Check sheet for the modelled part. Datum: model origin and axes. Units: mm. A direction names the side the tool comes from. Coordinates: 2 decimals unless noted, no trailing zeros. Write each loop counter-clockwise with the first axis right and the second up, starting at its lowest first coordinate (ties: lowest second). Pieces come first, ordered by that corner, then holes. Notation, with made-up numbers: (18, 65) - (34, 65) arc R22 cw to (34, 98) - close; hole circle Ø1 at (46, 31.5). An arc over 180 degrees is marked (long way). Use one line per item in the form item = value. Start each with the question number.
1. Tool access check on faces 1 (the face through (-26, -26, 25)), 2 (the face through (-38, 24.325, 30)), 3 (the face through (-17.54, 37, 30)), 4 (the face through (-26, -30.675, 12)). Record the directions out of +Z, -Z, +X, -X, +Y, -Y that give a thin tool (end or side, any length) a straight path to the whole face; none if there is none.
2. Cross-section at D-D on x = -19. Record the boundary of the cut face in (y, z), then the cut area to 3 significant figures.
3. Draft check along Z on faces 5 (the face through (-26, -26, 35)), 6 (the face through (-0.54, 9, 30)), 7 (the face through (-26, -8, 60)). Enter one of: +Z half, -Z half, draft (parallel to the pull), parting line (faces both ways), or undercut.
4. Go/stop test with a flat-tipped pin: pin 1 Ø11 at (x, z) = (-29, 31.5) entering from -Y. Record where the tip stops, or that it passes through.
5. Cross-section at B-B on x = -35. Record the boundary of the cut face in (y, z).
6. Cross-section at C-C on z = 51.5. Record the boundary of the cut face in (x, y).
7. Cross-section at A-A on y = 27.5. Record the boundary of the cut face in (x, z).
8. Scan lines: line 1 along Y through (x, z) = (-16, 15); line 2 along X through (y, z) = (21.5, 43.5); line 3 along Z through (x, y) = (-14.5, -22.5). Record each from-to range of solid material in increasing order.
```python
from build123d import *

# Parameters (mm, degrees)
BOSS_EXTRUDE2_DEPTH = 60
SKETCH2_W           = 10
SKETCH2_H           = 10
CUT_EXTRUDE1_DEPTH  = 60


with BuildPart() as part:
    # Sketch1 → Boss-Extrude2 (new body)
    with BuildSketch(Plane.XY):
        Polygon((-50.540381022, -30.675149326), (-0.540381022, -30.675149326), (-0.540381022, 49.324850674), (-17.540381022, 49.324850674), (-17.540381022, 24.324850674), (-8.540381022, 24.324850674), (-8.540381022, -5.675149326), (-42.540381022, -5.675149326), (-42.540381022, 24.324850674), (-33.540381022, 24.324850674), (-33.540381022, 49.324850674), (-50.540381022, 49.324850674), align=None)
    extrude(amount=BOSS_EXTRUDE2_DEPTH)

    # Sketch2 → Cut-Extrude1 (cut)
    with BuildSketch(Plane.ZY.offset(50.540381022)):
        with Locations((30, -25.675149326)):
            Rectangle(SKETCH2_W, SKETCH2_H)
    extrude(amount=-CUT_EXTRUDE1_DEPTH, mode=Mode.SUBTRACT)


solid = part.part
```
Final values:
q1.face_1 = +X, -X, -Y
q1.face_2 = +Z, -Z
q1.face_3 = +Z, -Z, +Y
q1.face_4 = +Z, -Z, +X, -X, -Y
q2.outline = (-30.68, 0) - (-5.68, 0) - (-5.68, 60) - (-30.68, 60) - (-30.68, 35) - (-20.68, 35) - (-20.68, 25) - (-30.68, 25) - close
q2.area = 1,400 mm²
q3.face_5 = undercut
q3.face_6 = draft
q3.face_7 = +Z half
q4.pin_1 = -30.68
q5.outline = (-30.68, 0) - (-5.68, 0) - (-5.68, 60) - (-30.68, 60) - (-30.68, 35) - (-20.68, 35) - (-20.68, 25) - (-30.68, 25) - close; (24.32, 0) - (49.32, 0) - (49.32, 60) - (24.32, 60) - close
q6.outline = (-50.54, -30.68) - (-0.54, -30.68) - (-0.54, 49.32) - (-17.54, 49.32) - (-17.54, 24.32) - (-8.54, 24.32) - (-8.54, -5.68) - (-42.54, -5.68) - (-42.54, 24.32) - (-33.54, 24.32) - (-33.54, 49.32) - (-50.54, 49.32) - close
q7.outline = (-50.54, 0) - (-33.54, 0) - (-33.54, 60) - (-50.54, 60) - close; (-17.54, 0) - (-0.54, 0) - (-0.54, 60) - (-17.54, 60) - close
q8.line_1 = -30.68 to -5.68, 24.32 to 49.32
q8.line_2 = -50.54 to -42.54, -8.54 to -0.54
q8.line_3 = 0 to 25, 35 to 60
